```python
from build123d import *

# Parameters (mm, degrees)
SKETCH_1_W      = 135.554325902
SKETCH_1_H      = 68.857107744
SKETCH_1_W_2    = 33.748913088
SKETCH_1_H_2    = 4
SKETCH_1_W_3    = 40
SKETCH_1_H_3    = 3
EXTRUDE_1_DEPTH = 4


with BuildPart() as part:
    # 草图1 → 凸台-拉伸1 (new body)
    with BuildSketch(Plane.XY):
        with Locations((62.437378831, 12.363507084)):
            Rectangle(SKETCH_1_W, SKETCH_1_H)
        with BuildLine():
            Line((7.008200879, 30.085320336), (12.008200879, 30.085320336))
            ThreePointArc((12.008200879, 30.085320336), (13.758200879, 28.335320336), (12.008200879, 26.585320336))
            Line((12.008200879, 26.585320336), (7.008200879, 26.585320336))
            ThreePointArc((7.008200879, 26.585320336), (5.258200879, 28.335320336), (7.008200879, 30.085320336))
        make_face(mode=Mode.SUBTRACT)
        with BuildLine():
            Line((39.008200879, 26.585320336), (34.008200879, 26.585320336))
            ThreePointArc((34.008200879, 26.585320336), (32.258200879, 28.335320336), (34.008200879, 30.085320336))
            Line((34.008200879, 30.085320336), (39.008200879, 30.085320336))
            ThreePointArc((39.008200879, 30.085320336), (40.758200879, 28.335320336), (39.008200879, 26.585320336))
        make_face(mode=Mode.SUBTRACT)
        with BuildLine():
            Line((7.008200879, -1.514679664), (12.008200879, -1.514679664))
            ThreePointArc((12.008200879, -1.514679664), (13.758200879, -3.264679664), (12.008200879, -5.014679664))
            Line((12.008200879, -5.014679664), (7.008200879, -5.014679664))
            ThreePointArc((7.008200879, -5.014679664), (5.258200879, -3.264679664), (7.008200879, -1.514679664))
        make_face(mode=Mode.SUBTRACT)
        with Locations((19.943744335, 20.535320336)):
            Rectangle(SKETCH_1_W_2, SKETCH_1_H_2, mode=Mode.SUBTRACT)
        with BuildLine():
            Line((39.008200879, -5.014679664), (34.008200879, -5.014679664))
            ThreePointArc((34.008200879, -5.014679664), (32.258200879, -3.264679664), (34.008200879, -1.514679664))
            Line((34.008200879, -1.514679664), (39.008200879, -1.514679664))
            ThreePointArc((39.008200879, -1.514679664), (40.758200879, -3.264679664), (39.008200879, -5.014679664))
        make_face(mode=Mode.SUBTRACT)
        with Locations((19.943744335, 4.535320336)):
            Rectangle(SKETCH_1_W_2, SKETCH_1_H_2, mode=Mode.SUBTRACT)
        with Locations((92.829401098, 20.435320336)):
            Rectangle(SKETCH_1_W_3, SKETCH_1_H_2, mode=Mode.SUBTRACT)
        with Locations((92.829401098, 7.335320336)):
            Rectangle(SKETCH_1_W_3, SKETCH_1_H_3, mode=Mode.SUBTRACT)
    extrude(amount=EXTRUDE_1_DEPTH)


solid = part.part
```
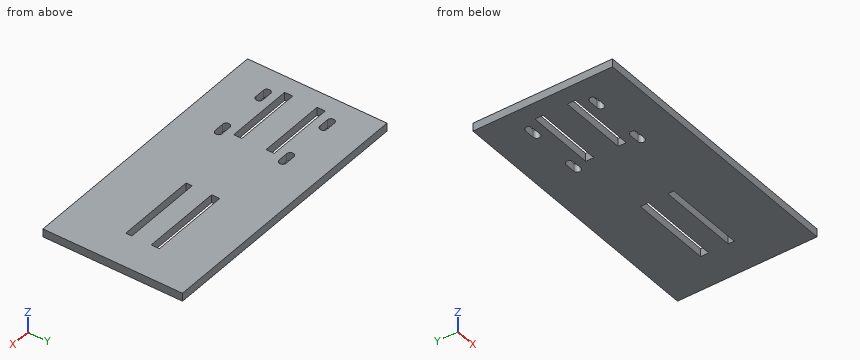
Could you check a few things on this model? Use its own coordinates, in mm. Round coordinates to 2 decimals unless told otherwise and drop trailing zeros. Write each loop counter-clockwise with the first axis right and the second up, starting at its lowest first coordinate (ties: lowest second). Pieces come first, ordered by that corner, then holes. Notation, with made-up numbers: M -30,89.25 L 18,89.25 A20 cw 18,128.25 Z; hole C -5,55.5 d2. An arc over 180 degrees is marked long. Write each question's results on one line, items separated by ' | '. Start each with the question number.
1. Imagine slicing it at A-A on x = 77. List the corners of the cut face in (y, z) for me, and give its area (3 significant figures).
2. Imagine slicing it at B-B on x = 24.5. List the corners of the cut face in (y, z) for me, and give its area (3 significant figures).
3. Imagine slicing it at C-C on z = 3.25. Count the separate pieces of the cut face and the enclosed holes in it, and give its area (3 significant figures).
4. I need wall thicknesses on L1, parallel to Y at x = 110.5, z = 1.35; L2, parallel to X at y = 20, z = 1.15; L3, parallel to Y at x = 28, z = 2.15. Which ranges of each line are inside material? Lowest first, please. Write a range as from..to.
Result sheet:
1) outline: M -22.07,0 L 5.84,0 L 5.84,4 L -22.07,4 Z; M 8.84,0 L 18.44,0 L 18.44,4 L 8.84,4 Z; M 22.44,0 L 46.79,0 L 46.79,4 L 22.44,4 Z | area: 247 mm^2
2) outline: M -22.07,0 L 2.54,0 L 2.54,4 L -22.07,4 Z; M 6.54,0 L 18.54,0 L 18.54,4 L 6.54,4 Z; M 22.54,0 L 46.79,0 L 46.79,4 L 22.54,4 Z | area: 243 mm^2
3) separate pieces: 1 | enclosed holes: 8 | area: 8,680 mm^2
4) L1: y = -22.07..5.84, 8.84..18.44, 22.44..46.79 | L2: x = -5.34..3.07, 36.82..72.83, 112.83..130.21 | L3: y = -22.07..2.54, 6.54..18.54, 22.54..46.79
